Drawing for the job (mm, zero at the part's lowest x, y, z). A direction names the side the tool comes from. Round coordinates to 2 decimals unless told otherwise and drop trailing zeros. Write each loop counter-clockwise with the first axis right and the second up, starting at its lowest first coordinate (ties: lowest second). Pieces come first, ordered by that corner, then holes. Notation, with made-up numbers: (83, -24.5) -> (126, -24.5) arc R16 ccw to (126, 2.5) -> close; hole circle Ø10 at (63.25, 47). An arc over 180 degrees is marked (long way). One line per question, with ' | ' between items.
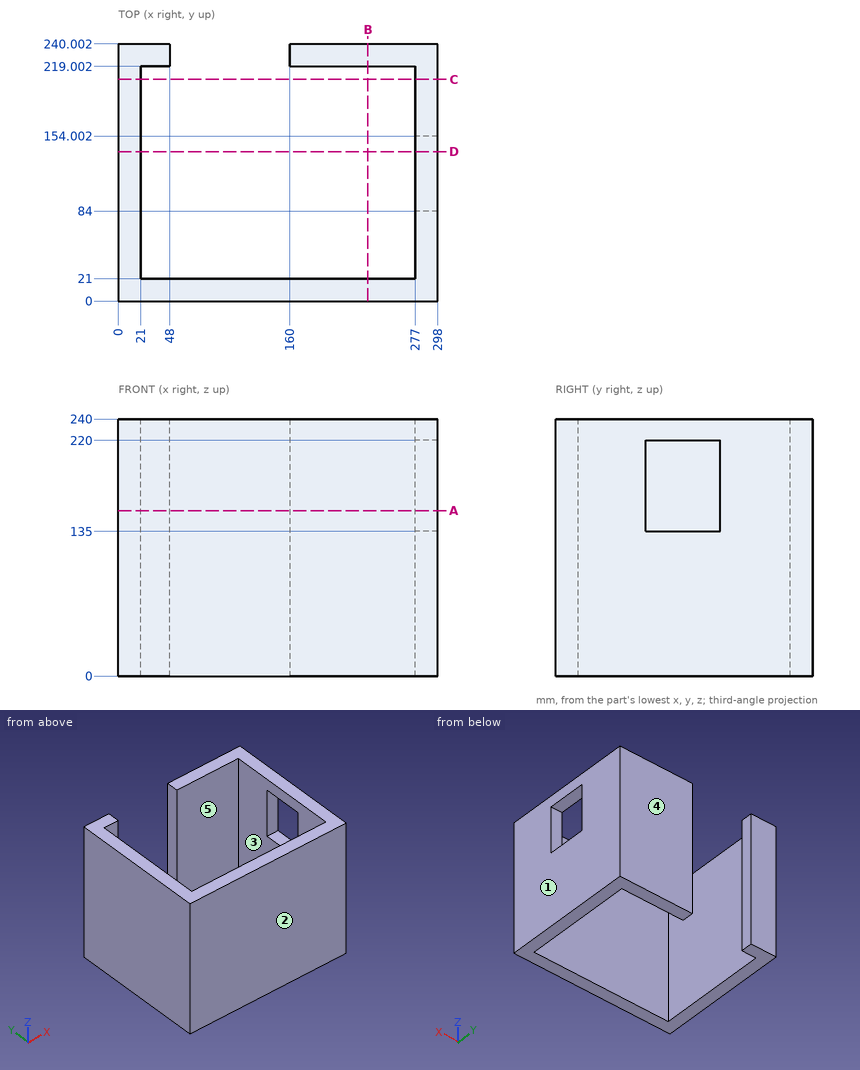
(1) Mould opens along X. For the marked faces 1, 2 and 3 say: pulls with the +X half, pulls with the -X half, needs draft (parallel to the pull), parting line crosses it, or undercut.
Calculated:
face 1: pulls with the +X half | face 2: needs draft | face 3: undercut
(2) Slice it at B-B (x = 233). Write the cut outline in (y, z), then the cut area to 3 significant figures.
Calculated:
outline: (0, 0) -> (21, 0) -> (21, 240) -> (0, 240) -> close; (219, 0) -> (240, 0) -> (240, 240) -> (219, 240) -> close | area: 10,100 mm2
(3) Drop flat-ended pins along their axis: pin 1 (6.5 mm diameter, centred on x = 291, z = 167, fed in from -Y); pin 2 (8 mm diameter, centred on x = 65, z = 46.5, fed in from +Y); pin 3 (6 mm diameter, centred on y = 131, z = 206.5, fed in from +X). Give the stop position or say it passes through.
Calculated:
pin 1: y = 0 | pin 2: y = 21 | pin 3: x = 21
(4) Slice it at D-D (y = 139.5). Write the cut outline in (x, z), then the cut area to 4 significant figures.
Calculated:
outline: (0, 0) -> (21, 0) -> (21, 240) -> (0, 240) -> close; (277, 0) -> (298, 0) -> (298, 135) -> (277, 135) -> close; (277, 220) -> (298, 220) -> (298, 240) -> (277, 240) -> close | area: 8,295 mm2
(5) Slice it at A-A (z = 154.5). Write the cut outline in (x, y).
Calculated:
outline: (0, 0) -> (298, 0) -> (298, 84) -> (277, 84) -> (277, 21) -> (21, 21) -> (21, 219) -> (48, 219) -> (48, 240) -> (0, 240) -> close; (160, 219) -> (277, 219) -> (277, 154) -> (298, 154) -> (298, 240) -> (160, 240) -> close
(6) Wall check: line 1 (X direction, y = 78, z = 142.5); line 2 (Y direction, x = 266.5, z = 190); line 3 (X direction, y = 90, z = 215). Give the ranges that are in metal, low to high. Write a range as from..to.
Calculated:
line 1: 0..21, 277..298 | line 2: 0..21, 219..240 | line 3: 0..21
(7) Slice it at C-C (y = 207). Write the cut outline in (x, z).
Calculated:
outline: (0, 0) -> (21, 0) -> (21, 240) -> (0, 240) -> close; (277, 0) -> (298, 0) -> (298, 240) -> (277, 240) -> close
(8) 3-axis set-ups, long thin cutter, end or side, ignore diameter. For the marked faces 4 and 5: which of +Z, -Z, +X, -X, +Y, -Y reach the whole face in a straight line?
Calculated:
face 4: +Z, -Z, +X, -X, +Y | face 5: +Z, -Z
